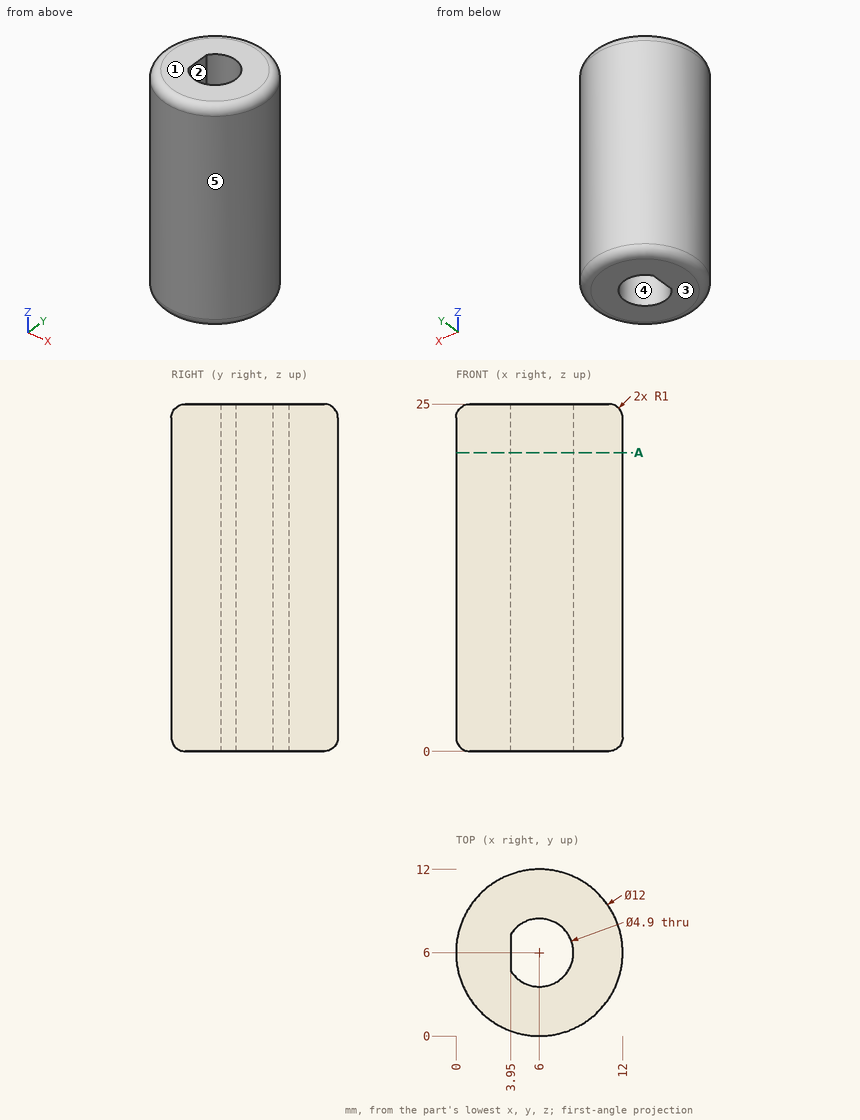
Study the drawing (mm; zero at the part's minimum x, y, z) and answer. A direction names the side the tool comes from. Round coordinates to 2 decimals unless told otherwise and drop trailing zeros. Write each loop counter-clockwise with the first axis right and the second up, starting at its lowest first coordinate (ties: lowest second). Pieces come first, ordered by that corner, then holes. Notation, with made-up numbers: (80.25, 11) -> (100.25, 11) arc R21 cw to (100.25, 22) -> close; hole circle Ø9 at (-27.5, 29). An arc over 180 degrees is marked (long way). Write item = value, one per line.
1) Which of the six approach directions +Z, -Z, +X, -X, +Y, -Y give full straight-line access (tool end or side, diameter ignored) to the marked faces 1 and 2?
Check values:
face_1 = +Z, +X, -X, +Y, -Y
face_2 = +Z, -Z
2) For a pull along Y with two mould halves and no side action, classify the marked faces 3, 4 and 5 as released by +Y, released by -Y, zero draft, split by the parting line, or undercut.
Check values:
face_3 = zero draft
face_4 = undercut
face_5 = split by the parting line
3) Section A-A on z = 21.5 is taken. Write down the section's boundary in (x, y).
Check values:
outline = circle Ø12 at (6, 6); hole (3.95, 4.66) arc R2.45 ccw (long way) to (3.95, 7.34) -> close
4) Given pin 1 (5 mm diameter, centred on y = 2, z = 5, fed in from -X); pin 2 (5 mm diameter, centred on y = 9.5, z = 20, fed in from -X); pin 3 (6 mm diameter, centred on y = 2.5, z = 8, fed in from -X), each flat-ended and moving along its own axis, determine where each tip first touches the part or whether it passes through.
Check values:
pin_1 = 0.19
pin_2 = 0.08
pin_3 = 0.02
5) Straight lines are drawn through the part: line 1 along Y through (x, z) = (6, 16.25); line 2 along Z through (x, y) = (7.75, 10.75); line 3 along X through (y, z) = (3.75, 21). For each, find the intervals that lie inside material, in ascending order. Write a range as [from, to].
Check values:
line_1 = [0, 3.55], [8.45, 12]
line_2 = [0, 25]
line_3 = [0.44, 5.03], [6.97, 11.56]
